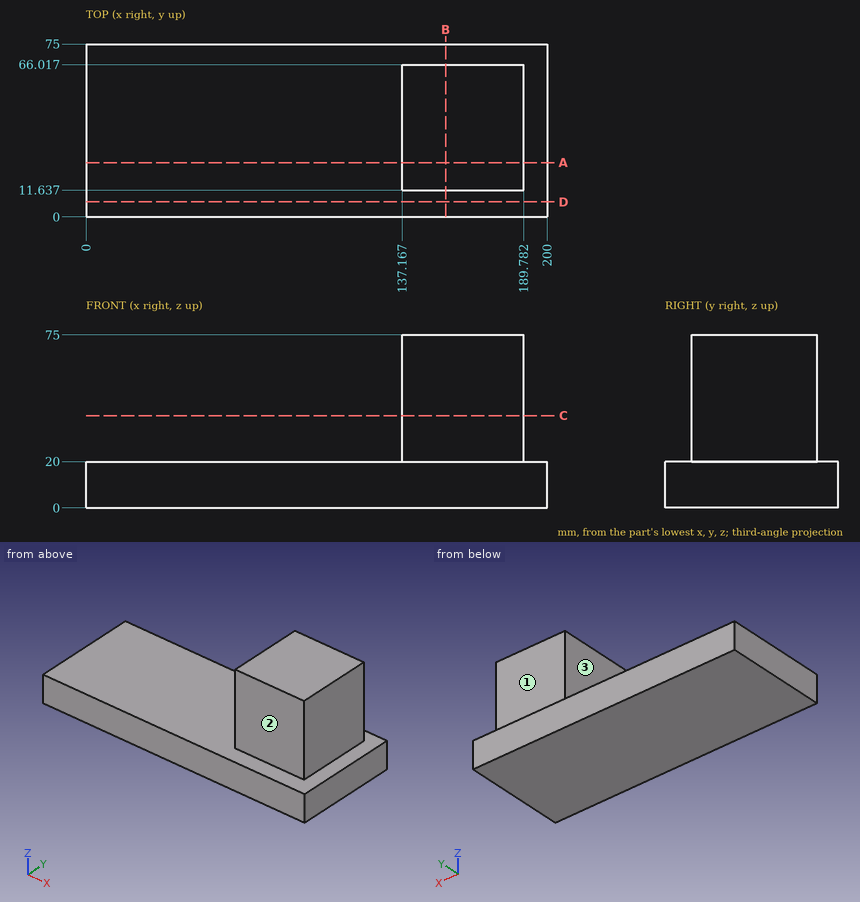
Could you check a few things on this drawing? It's one solid part, dimensions in mm from its lowest x, y, z. A direction names the side the tool comes from. Coordinates: 2 decimals unless noted, no trailing zeros. Order: outer loops, then holes, each group sorted by start corner. A loop starts at its lowest first (then second) coordinate and runs counter-clockwise, first axis right, second up. Notation, with made-up numbers: M 4,68 L 39,68 A27 ccw 39,99 Z; hole C 79,29.5 d3. An arc over 180 degrees is marked long. Answer as a JSON object with one key per item and string values. Group by question number.
(1) Which directions (+Z, -Z, +X, -X, +Y, -Y) give clear straight access to the entire face, cutting with the end or side of a thin tool? Please do the marked faces 1, 2 and 3.
(2) I need wall thicknesses on probe 1 along Y at (x, z) = (166.5, 42); probe 2 along X at (y, z) = (32, 51); probe 3 along Z at (x, y) = (136, 45.5). Which ranges of each line are inside material? Lowest first, please.
(3) Suppose I cut it at A-A, the plane y = 23.5. Please give me the cut outline in (x, z), then the cut area to 3 significant figures.
(4) For pin 1 (10 mm diameter, centred on y = 51.5, z = 56.5, fed in from +X); pin 2 (16.5 mm diameter, centred on y = 50.5, z = 36.5, fed in from -X); pin 3 (3 mm diameter, centred on x = 168.5, z = 62.5, fed in from -Y), each with a flat end and sliding along its axis, tell me the tip position at first contact or that it passes through.
(5) Suppose I cut it at D-D, the plane y = 6.5. Please give me the cut outline in (x, z).
(6) Suppose I cut it at C-C, the plane z = 40. Please give me the cut outline in (x, y).
(7) Suppose I cut it at B-B, the plane x = 156. Please give me the cut outline in (y, z).
Values found:
{
 "1": {"face 1": "+Z, +X, -X, +Y", "face 2": "+Z, +X, -X, -Y", "face 3": "+Z, -X, +Y, -Y"},
 "2": {"probe 1": "y = 11.64 to 66.02", "probe 2": "x = 137.17 to 189.78", "probe 3": "z = 0 to 20"},
 "3": {"outline": "M 0,0 L 200,0 L 200,20 L 189.78,20 L 189.78,75 L 137.17,75 L 137.17,20 L 0,20 Z", "area": "6,890 mm^2"},
 "4": {"pin 1": "stops at x = 189.78", "pin 2": "stops at x = 137.17", "pin 3": "stops at y = 11.64"},
 "5": {"outline": "M 0,0 L 200,0 L 200,20 L 0,20 Z"},
 "6": {"outline": "M 137.17,11.64 L 189.78,11.64 L 189.78,66.02 L 137.17,66.02 Z"},
 "7": {"outline": "M 0,0 L 75,0 L 75,20 L 66.02,20 L 66.02,75 L 11.64,75 L 11.64,20 L 0,20 Z"}
}
